CAD build for the part. Positions are in the model's coordinates, mm. A direction names the side the tool comes from. Round coordinates to 2 decimals unless told otherwise and drop trailing zeros. Loops run counter-clockwise (first coordinate to the right, second up) from the corner with the lowest first, then second, coordinate; pieces in that order, holes last. Notation, with made-up numbers: M -35,77 L 5,77 A21 cw 5,103 Z; hole C 40,26 d9. An arc over 180 degrees is marked long. Use a Markdown table: item, result. Add a question column.
(1) Wall check: L1, parallel to X at y = -12.5, z = 21.5; L2, parallel to Y at x = 60, z = 22; L3, parallel to X at y = -20.75, z = 23.5. Give the ranges that are in metal, low to high.
(2) Which spindle directions (+Z, -Z, +X, -X, +Y, -Y) get a long thin tool onto all of the face, cutting with end or side? Do faces 5 (the face through (50.832, -12.325, 39.565)), 6 (the face through (0, -12, 44.9)), 7 (the face through (53.257, -12.797, 30.464)). Say none if no direction does.
(3) Two-plate mould, pull along Y, no slides. Class faces 1 (the face through (-71.297, -23.859, 26.328)), 2 (the face through (71.297, -1.141, 26.164)), 3 (the face through (30.4, -12.3, 35.1)), 4 (the face through (-60, -8, 25.4)): released by +Y, released by -Y, zero draft, split by the parting line, or undercut.
(4) Band-saw the part on C-C, the plane x = 60. Write the cut outline in (y, z), and give its area (3 significant figures).
(5) Band-saw the part on A-A, the plane z = 28.5. Write the cut outline in (x, y).
(6) Flat gauge pins, fed straight in: P1, Ø14, axis at x = -60, y = -12.5, coming from the +Z side; P2, Ø15, axis at x = -57, y = -11, coming from the +Z side; P3, Ø7, axis at x = 57, y = -15.5, coming from the +Z side. Where does each tip first touch, or does it go through?
(7) Band-saw the part on D-D, the plane x = 7.5. Write the cut outline in (y, z).
(8) Band-saw the part on B-B, the plane y = -10.75. Give the number of separate pieces and of enclosed holes in the cut face, and give its area (3 significant figures).
from build123d import *

# Parameters (mm, degrees)
PAD_DEPTH       = 25
SKETCH001_R     = 4.3
POCKET_DEPTH    = 29.501
SKETCH002_R     = 6.75
POCKET001_DEPTH = 24.501
FILLET_R        = 4
FILLET001_R     = 18


with BuildPart() as part:
    # Sketch → Pad (new body)
    with BuildSketch(Plane.XZ):
        with BuildLine():
            ThreePointArc((-40.4, 30.9), (-30.500505, 35.000505), (-26.4, 44.9))
            Line((-26.4, 44.9), (26.4, 44.9))
            ThreePointArc((26.4, 44.9), (30.500505, 35.000505), (40.4, 30.9))
            Line((40.4, 20.4), (40.4, 30.9))
            Line((72.5, 20.4), (40.4, 20.4))
            Line((72.5, 30.4), (72.5, 20.4))
            Line((26.4, 49.9), (72.5, 30.4))
            Line((-26.4, 49.9), (26.4, 49.9))
            Line((-72.5, 30.4), (-26.4, 49.9))
            Line((-72.5, 20.4), (-72.5, 30.4))
            Line((-40.4, 20.4), (-72.5, 20.4))
            Line((-40.4, 30.9), (-40.4, 20.4))
        make_face()
    extrude(amount=PAD_DEPTH)

    # Sketch001 (on Face11 of Pad) → Pocket (cut, through all)
    with BuildSketch(Plane(origin=(0, 0, 20.4), x_dir=(1, 0, 0), z_dir=(0, 0, -1))):
        with Locations((-60, 12.5)):
            Circle(SKETCH001_R)
        with Locations((60, 12.5)):
            Circle(SKETCH001_R)
    extrude(amount=-POCKET_DEPTH, mode=Mode.SUBTRACT)

    # Sketch002 (on Face6 of Pocket) → Pocket001 (cut, through all)
    with BuildSketch(Plane(origin=(0, 0, 25.4), x_dir=(1, 0, 0), z_dir=(0, 0, -1))):
        with Locations((-60, 12.5)):
            Circle(SKETCH002_R)
        with Locations((60, 12.5)):
            Circle(SKETCH002_R)
    extrude(amount=-POCKET001_DEPTH, mode=Mode.SUBTRACT)

    # Fillet
    fillet_edges = [part.edges().sort_by_distance(p)[0] for p in [
        (-72.5, -25, 25.4),
        (-72.5, 0, 25.4),
        (72.5, -25, 25.4),
        (72.5, 0, 25.4),
    ]]
    fillet(fillet_edges, radius=FILLET_R)

    # Fillet001
    fillet001_edges = [part.edges().sort_by_distance(p)[0] for p in [
        (-26.4, -12.5, 49.9),
        (26.4, -12.5, 49.9),
    ]]
    fillet(fillet001_edges, radius=FILLET001_R)


solid = part.part
Return value:
| question | item | result |
|---|---|---|
| 1 | L1 | -72.5 to -64.3, -55.7 to -40.4, 40.4 to 55.7, 64.3 to 72.5 |
| 1 | L2 | -25 to -16.8, -8.2 to 0 |
| 1 | L3 | -72.5 to -40.4, 40.4 to 72.5 |
| 2 | face 5 | +Z, +X, +Y, -Y |
| 2 | face 6 | -Z, +Y, -Y |
| 2 | face 7 | +Z |
| 3 | face 1 | released by -Y |
| 3 | face 2 | released by +Y |
| 3 | face 3 | zero draft |
| 3 | face 4 | undercut |
| 4 | outline | M -25,20.4 L -16.8,20.4 L -16.8,25.4 L -19.25,25.4 L -19.25,35.69 L -25,35.69 Z; M -8.2,20.4 L 0,20.4 L 0,35.69 L -5.75,35.69 L -5.75,25.4 L -8.2,25.4 Z |
| 4 | area | 200 mm^2 |
| 5 | outline | M -72.5,-21 A4 ccw -68.5,-25 L -40.4,-25 L -40.4,0 L -68.5,0 A4 ccw -72.5,-4 Z; M 40.4,-25 L 68.5,-25 A4 ccw 72.5,-21 L 72.5,-4 A4 ccw 68.5,0 L 40.4,0 Z; hole C -60,-12.5 d13.5; hole C 60,-12.5 d13.5 |
| 6 | P1 | z = 38.65 |
| 6 | P2 | z = 40.13 |
| 6 | P3 | z = 38.44 |
| 7 | outline | M -25,44.9 L 0,44.9 L 0,49.9 L -25,49.9 Z |
| 8 | separate pieces | 3 |
| 8 | enclosed holes | 0 |
| 8 | area | 1,360 mm^2 |
